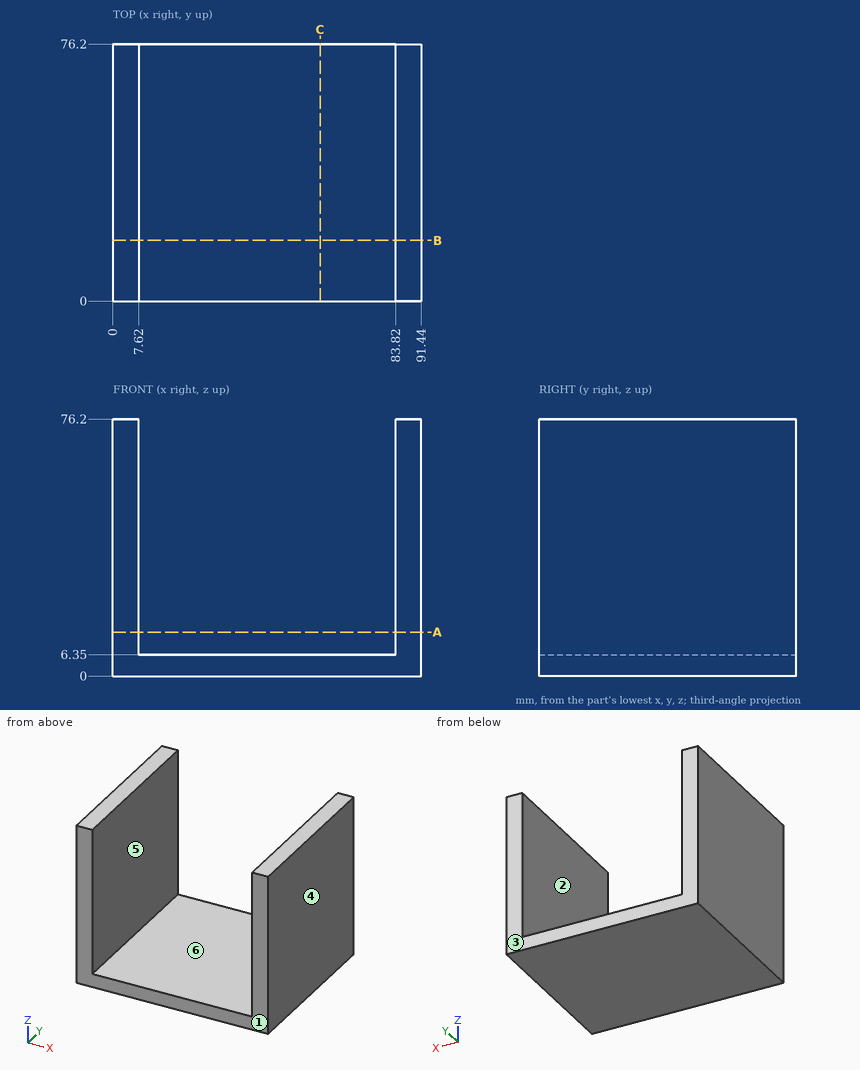
Study the drawing (mm; zero at the part's minimum x, y, z) and answer. A direction names the side the tool comes from. Round coordinates to 2 decimals unless told otherwise and drop trailing zeros. Write each loop counter-clockwise with the first axis right and the second up, starting at its lowest first coordinate (ties: lowest second). Pieces come first, ordered by that corner, then holes. Notation, with made-up numbers: (0.5, 31) -> (7.5, 31) arc R17 ccw to (7.5, 51) -> close; hole circle Ø7 at (85.25, 43). An arc over 180 degrees is marked (long way). Use CSV: the item, a comma, the result in double quotes. Start each with the question number.
(1) Each of these flat-tipped pins is pushed along its axis until it touches: pin 1 (10 mm diameter, centred on x = 17, y = 32, fed in from +Z); pin 2 (5 mm diameter, centred on x = 80.5, z = 14.5, fed in from -Y). Where does it stop, or does it pass through?
(2) Which of the six approach directions +Z, -Z, +X, -X, +Y, -Y give full straight-line access (tool end or side, diameter ignored) to the marked faces 1 and 2?
(3) Section B-B on y = 18 is taken. Give the vertices of the cut face in (x, z), then the cut area to 3 significant figures.
(4) Section A-A on z = 13 is taken. Give the vertices of the cut face in (x, y), then the cut area to 3 significant figures.
(5) Section C-C on x = 61.5 is taken. Give the vertices of the cut face in (y, z), then the cut area to 3 significant figures.
(6) The mould has two halves that part along X. Classify the marked faces 3, 4, 5 and 6: released by +X, released by -X, zero draft, split by the parting line, or undercut.
(7) Consider L1, parallel to X at y = 62, z = 39; L2, parallel to Z at x = 40.5, y = 10. Determine where each line is inside the solid, lowest interval first. Write a range as from..to.
A:
1,pin 1,"stops at z = 6.35"
1,pin 2,"passes through"
2,face 1,"+Z, -Z, +X, -X, -Y"
2,face 2,"+Z, +Y, -Y"
3,outline,"(0, 0) -> (91.44, 0) -> (91.44, 76.2) -> (83.82, 76.2) -> (83.82, 6.35) -> (7.62, 6.35) -> (7.62, 76.2) -> (0, 76.2) -> close"
3,area,"1,650 mm²"
4,outline,"(0, 0) -> (7.62, 0) -> (7.62, 76.2) -> (0, 76.2) -> close; (83.82, 0) -> (91.44, 0) -> (91.44, 76.2) -> (83.82, 76.2) -> close"
4,area,"1,160 mm²"
5,outline,"(0, 0) -> (76.2, 0) -> (76.2, 6.35) -> (0, 6.35) -> close"
5,area,"484 mm²"
6,face 3,"zero draft"
6,face 4,"released by +X"
6,face 5,"undercut"
6,face 6,"undercut"
7,L1,"x = 0..7.62, 83.82..91.44"
7,L2,"z = 0..6.35"
